Build history of the part. All positions in model axes, mm. Face numbers are marked on the shaded views. Give positions to 0.01 mm unless a question says otherwise; leave off trailing zeros. Order: outer loops, then holes, each group sorted by start corner. A loop starts at its lowest first (then second) coordinate and runs counter-clockwise, first axis right, second up. Notation, with made-up numbers: (54, 42.5) - (112, 42.5) arc R27 ccw to (112, 58.5) - close; hole circle Ø7 at (58.25, 39.5). An arc over 180 degrees is marked (long way). One line per item, written item: value.
```python
from build123d import *

# Parameters (mm, degrees)
SKETCH1_R           = 12.5
SKETCH1_R_2         = 1.75
SKETCH1_R_3         = 3.75
BOSS_EXTRUDE1_DEPTH = 4
CHAMFER2_SIZE       = 1.2


with BuildPart() as part:
    # Sketch1 → Boss-Extrude1 (new body)
    with BuildSketch(Plane.XY):
        with Locations((30.875, 0)):
            Circle(SKETCH1_R)
        with Locations((30.875, 8.5)):
            Circle(SKETCH1_R_2, mode=Mode.SUBTRACT)
        with Locations((30.875, -8.5)):
            Circle(SKETCH1_R_2, mode=Mode.SUBTRACT)
        with Locations((30.875, 0)):
            Circle(SKETCH1_R_3, mode=Mode.SUBTRACT)
    extrude(amount=BOSS_EXTRUDE1_DEPTH)

    # Chamfer2
    chamfer2_edges = [part.edges().sort_by_distance(p)[0] for p in [
        (29.125, 8.5, 4),
        (29.125, -8.5, 4),
    ]]
    chamfer(chamfer2_edges, length=CHAMFER2_SIZE)


solid = part.part
```
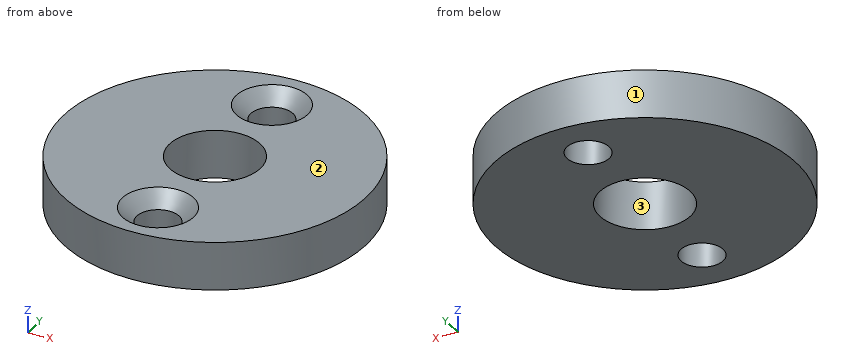
(1) Pull direction Y, two halves, no side cores. Call the marked faces 1, 2 and 3: +Y half, -Y half, draft (parallel to the pull), parting line (faces both ways), or undercut.
Completed:
face 1: parting line
face 2: draft
face 3: undercut
(2) Slice it at D-D, the plane x = 23.5. Give the cut face in (y, z), and give its area (3 significant figures).
Completed:
outline: (-10.09, 0) - (10.09, 0) - (10.09, 4) - (-10.09, 4) - close
area: 80.7 mm²
(3) Slice it at B-B, the plane z = 1.8. Give the cut face in (x, y) (3 decimals), and give its area (3 significant figures).
Completed:
outline: circle Ø25 at (30.875, 0); hole circle Ø7.5 at (30.875, 0); hole circle Ø3.5 at (30.875, -8.5); hole circle Ø3.5 at (30.875, 8.5)
area: 427 mm²
(4) Slice it at C-C, the plane y = -8.5. Give the cut face in (x, z) (3 decimals), and give its area (3 significant figures).
Completed:
outline: (21.71, 0) - (29.125, 0) - (29.125, 2.8) - (27.925, 4) - (21.71, 4) - close; (32.625, 0) - (40.04, 0) - (40.04, 4) - (33.825, 4) - (32.625, 2.8) - close
area: 57.9 mm²
(5) Pin check, flat tips, straight feed: P1, Ø2, axis at x = 40.5, z = 2.5, coming from the +Y side; P2, Ø2, axis at x = 28.5, z = 2, coming from the +Y side. Stop position of each tip, or through.
Completed:
P1: y = 9.05
P2: y = 12.42
(6) Slice it at A-A, the plane y = 0. Give the cut face in (x, z) (3 decimals), and give its area (3 significant figures).
Completed:
outline: (18.375, 0) - (27.125, 0) - (27.125, 4) - (18.375, 4) - close; (34.625, 0) - (43.375, 0) - (43.375, 4) - (34.625, 4) - close
area: 70.0 mm²
(7) Drill centre lines: line 1 (Y direction, x = 31.75, z = 3.1); line 2 (Y direction, x = 30.5, z = 3); line 3 (X direction, y = -0.75, z = 0.65). Where is each one in solid material? Low to high.
Completed:
line 1: -12.47 to -10.35, -6.65 to -3.65, 3.65 to 6.65, 10.35 to 12.47
line 2: -12.49 to -10.41, -6.59 to -3.73, 3.73 to 6.59, 10.41 to 12.49
line 3: 18.4 to 27.2, 34.55 to 43.35
